Build history of the part. All positions in model axes, mm. A direction names the side the tool comes from. Round coordinates to 2 decimals unless told otherwise and drop trailing zeros. Write each loop counter-clockwise with the first axis right and the second up, starting at its lowest first coordinate (ties: lowest second). Pieces come first, ordered by that corner, then holes. Notation, with made-up numbers: M -6,-24 L 35,-24 A20 cw 35,11 Z; hole C 40,-16.75 d6. An arc over 180 degrees is marked long. Write item = value, one per line. Start each with the question number.
Q1. Band-saw the part on B-B on x = 58. Write the cut outline in (y, z).
Q2. Drop flat-ended pins along their axis: P1, Ø3, axis at y = 113, z = 1.5, coming from the +X side; P2, Ø1.9, axis at y = -114, z = 1.5, coming from the -X side; P3, Ø1.9, axis at x = -146.5, z = 4.5, coming from the -Y side. Give the stop position or say it passes through.
Q3. Tool access for faces 5 (the flat face through (66, 113, 3)), 6 (the flat face through (-146, -78, 3)), 7 (the flat face through (143, 84, 3)), 8 (the flat face through (6, -113, 3)): list every direction of +Z, -Z, +X, -X, +Y, -Y with a clear straight run to the whole face (end or side of a thin tool).
Q4. Band-saw the part on A-A on y = 86. Write the cut outline in (x, z), plus the area to 3 significant figures.
Q5. Probe L1, parallel to X at y = -57, z = 1.5; L2, parallel to Y at x = -136.5, z = 4. List the from-to ranges inside material, lowest first.
Q6. Pull direction X, two halves, no side cores. Call faces 1 (the flat face through (143, -12, 3)), 2 (the flat face through (36, -110, 3)), 3 (the flat face through (-143, -109, 3)), 4 (the flat face through (12, -110, 3)): released by +X, released by -X, zero draft, split by the parting line, or undercut.
```python
from build123d import *

# Parameters (mm, degrees)
F0_W     = 286
F0_H     = 220
F1_DEPTH = 6.2
F2_W     = 5
F2_H     = 6.2
F2_W_2   = 12
F3_DEPTH = 6.2
F4_W     = 6.2
F4_H     = 12
F5_DEPTH = 6.2


with BuildPart() as f1:
    # F0 (on Top) → F1 (new body)
    with BuildSketch(Plane.XY):
        Rectangle(F0_W, F0_H)
    extrude(amount=F1_DEPTH)

    # F2 (on face) → F3 (join, through all)
    with BuildSketch(Plane.XY.offset(6.2)):
        with Locations((140.5, 113.1)):
            Rectangle(F2_W, F2_H)
        with Locations((120, 113.1)):
            Rectangle(F2_W_2, F2_H)
        with Locations((96, 113.1)):
            Rectangle(F2_W_2, F2_H)
        with Locations((72, 113.1)):
            Rectangle(F2_W_2, F2_H)
        with Locations((48, 113.1)):
            Rectangle(F2_W_2, F2_H)
        with Locations((24, 113.1)):
            Rectangle(F2_W_2, F2_H)
        with Locations((0, 113.1)):
            Rectangle(F2_W_2, F2_H)
        with Locations((-24, 113.1)):
            Rectangle(F2_W_2, F2_H)
        with Locations((-48, 113.1)):
            Rectangle(F2_W_2, F2_H)
        with Locations((-72, 113.1)):
            Rectangle(F2_W_2, F2_H)
        with Locations((-96, 113.1)):
            Rectangle(F2_W_2, F2_H)
        with Locations((-120, 113.1)):
            Rectangle(F2_W_2, F2_H)
        with Locations((-140.5, 113.1)):
            Rectangle(F2_W, F2_H)
        with Locations((-140.5, -113.1)):
            Rectangle(F2_W, F2_H)
        with Locations((-120, -113.1)):
            Rectangle(F2_W_2, F2_H)
        with Locations((-96, -113.1)):
            Rectangle(F2_W_2, F2_H)
        with Locations((-72, -113.1)):
            Rectangle(F2_W_2, F2_H)
        with Locations((-48, -113.1)):
            Rectangle(F2_W_2, F2_H)
        with Locations((-24, -113.1)):
            Rectangle(F2_W_2, F2_H)
        with Locations((0, -113.1)):
            Rectangle(F2_W_2, F2_H)
        with Locations((24, -113.1)):
            Rectangle(F2_W_2, F2_H)
        with Locations((48, -113.1)):
            Rectangle(F2_W_2, F2_H)
        with Locations((72, -113.1)):
            Rectangle(F2_W_2, F2_H)
        with Locations((96, -113.1)):
            Rectangle(F2_W_2, F2_H)
        with Locations((120, -113.1)):
            Rectangle(F2_W_2, F2_H)
        with Locations((140.5, -113.1)):
            Rectangle(F2_W, F2_H)
    extrude(amount=-F3_DEPTH)

    # F4 (on face) → F5 (join, through all)
    with BuildSketch(Plane.XY.offset(6.2)):
        with Locations((146.1, -96)):
            Rectangle(F4_W, F4_H)
        with Locations((146.1, -72)):
            Rectangle(F4_W, F4_H)
        with Locations((146.1, -48)):
            Rectangle(F4_W, F4_H)
        with Locations((146.1, -24)):
            Rectangle(F4_W, F4_H)
        with Locations((146.1, 0)):
            Rectangle(F4_W, F4_H)
        with Locations((146.1, 24)):
            Rectangle(F4_W, F4_H)
        with Locations((146.1, 48)):
            Rectangle(F4_W, F4_H)
        with Locations((146.1, 72)):
            Rectangle(F4_W, F4_H)
        with Locations((146.1, 96)):
            Rectangle(F4_W, F4_H)
        with Locations((-146.1, 96)):
            Rectangle(F4_W, F4_H)
        with Locations((-146.1, 72)):
            Rectangle(F4_W, F4_H)
        with Locations((-146.1, 48)):
            Rectangle(F4_W, F4_H)
        with Locations((-146.1, 24)):
            Rectangle(F4_W, F4_H)
        with Locations((-146.1, 0)):
            Rectangle(F4_W, F4_H)
        with Locations((-146.1, -24)):
            Rectangle(F4_W, F4_H)
        with Locations((-146.1, -48)):
            Rectangle(F4_W, F4_H)
        with Locations((-146.1, -72)):
            Rectangle(F4_W, F4_H)
        with Locations((-146.1, -96)):
            Rectangle(F4_W, F4_H)
    extrude(amount=-F5_DEPTH)


solid = f1.part
```
Conclusion:
q1.outline = M -110,0 L 110,0 L 110,6.2 L -110,6.2 Z
q2.P1 = 143
q2.P2 = -143
q2.P3 = -102
q3.face_5 = +Z, -Z, +Y
q3.face_6 = +Z, -Z, -X
q3.face_7 = +Z, -Z, +X
q3.face_8 = +Z, -Z, -Y
q4.outline = M -143,0 L 143,0 L 143,6.2 L -143,6.2 Z
q4.area = 1,770 mm^2
q5.L1 = -143 to 143
q5.L2 = -110 to 110
q6.face_1 = released by +X
q6.face_2 = undercut
q6.face_3 = released by -X
q6.face_4 = undercut
